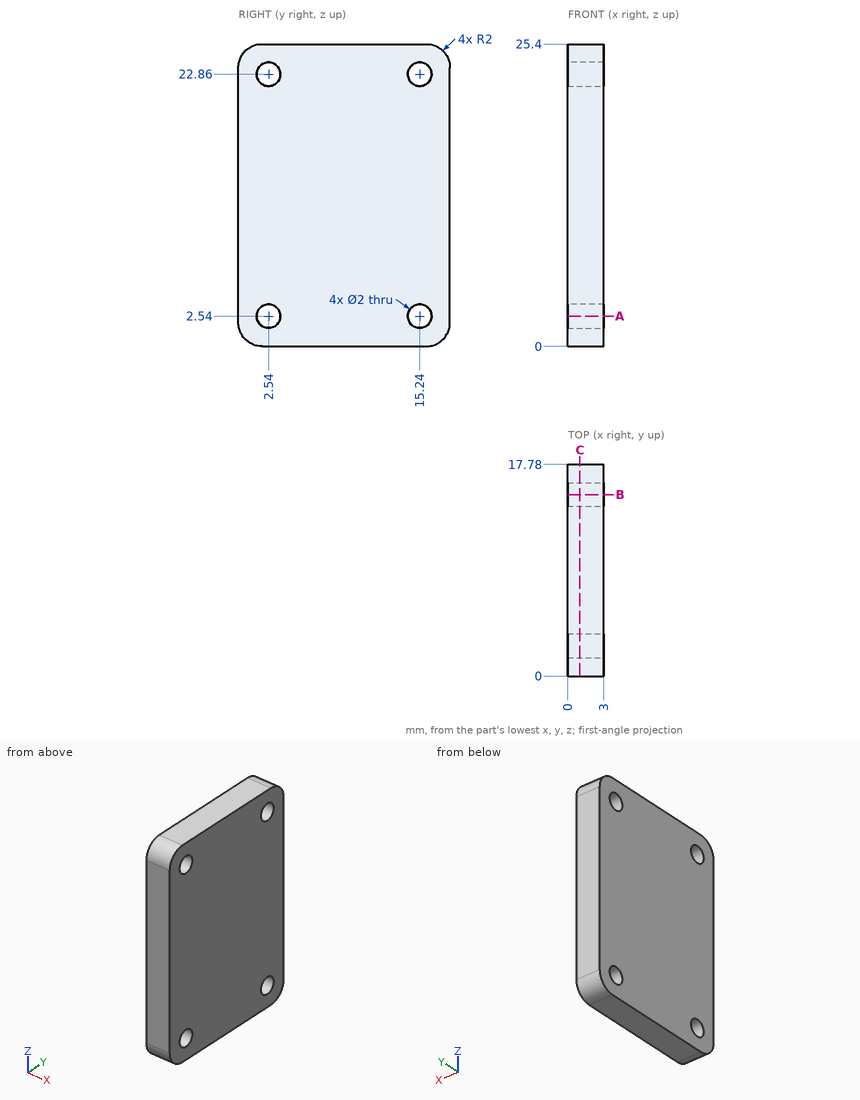
Answer from the drawing. Dimensions are ordinates in mm from the lowest x, y and z of the part. Give positions to 0.01 mm unless a question says otherwise; leave off trailing zeros. Order: outer loops, then holes, each group sorted by start corner. A loop starts at its lowest first (then second) coordinate and runs counter-clockwise, first axis right, second up. Notation, with made-up numbers: (64, 29) - (73, 29) arc R16 ccw to (73, 40) - close; hole circle Ø8 at (52, -15.5). An arc over 180 degrees is marked (long way). One line per item, written item: value. Start each with the question number.
1) Given pin 1 Ø2.5 at (y, z) = (2.54, 22.86) entering from +X, flat-ended and moving along its own axis, determine where the tip first touches the part or whether it passes through.
2) A cutting plane is placed at A-A on z = 2.54. Give the vertices of the cut face in (x, y), then the cut area to 3 significant figures.
3) Find the intervals of material crossed by L1, parallel to Y at x = 2.4, z = 2.54; L2, parallel to Z at x = 1.3, y = 15.25; L3, parallel to Z at x = 0.8, y = 1.75, in increasing order.
4) A cutting plane is placed at B-B on y = 15.24. Give the vertices of the cut face in (x, z), then the cut area to 3 significant figures.
5) A cutting plane is placed at C-C on x = 1. Give the vertices of the cut face in (y, z).
Answer sheet:
1. pin 1: stops at x = 3
2. outline: (0, 0) - (3, 0) - (3, 1.54) - (0, 1.54) - close; (0, 3.54) - (3, 3.54) - (3, 14.24) - (0, 14.24) - close; (0, 16.24) - (3, 16.24) - (3, 17.78) - (0, 17.78) - close
2. area: 41.3 mm2
3. L1: y = 0 to 1.54, 3.54 to 14.24, 16.24 to 17.78
3. L2: z = 0 to 1.54, 3.54 to 21.86, 23.86 to 25.4
3. L3: z = 0.02 to 1.93, 3.15 to 22.25, 23.47 to 25.38
4. outline: (0, 0) - (3, 0) - (3, 1.54) - (0, 1.54) - close; (0, 3.54) - (3, 3.54) - (3, 21.86) - (0, 21.86) - close; (0, 23.86) - (3, 23.86) - (3, 25.4) - (0, 25.4) - close
4. area: 64.2 mm2
5. outline: (0, 2) arc R2 ccw to (2, 0) - (15.78, 0) arc R2 ccw to (17.78, 2) - (17.78, 23.4) arc R2 ccw to (15.78, 25.4) - (2, 25.4) arc R2 ccw to (0, 23.4) - close; hole circle Ø2 at (2.54, 2.54); hole circle Ø2 at (2.54, 22.86); hole circle Ø2 at (15.24, 2.54); hole circle Ø2 at (15.24, 22.86)
